Input: part model. Units: mm. Frame: model coordinates. A direction names the side the tool comes from. Give positions to 0.01 mm unless a question says otherwise; leave off trailing zeros. Write each loop counter-clockwise with the first axis right and the second up, starting at its lowest first coordinate (ties: lowest second). Pieces come first, ordered by that corner, then holes. Notation, with made-up numbers: M 7.5,12 L 47.5,12 A31 cw 47.5,47 Z; hole C 63,12.25 d4. An arc over 180 degrees is marked long. Use CSV: the item, a comma, the result in double quotes. Start each with the question number.
from build123d import *

# Parameters (mm, degrees)
F2_R     = 14
F3_DEPTH = 25
F4_SIZE  = 1
F5_R     = 1


with BuildPart() as f1:
    # F0 (on Front) → F1 (revolve)
    with BuildSketch(Plane.XZ):
        Polygon((0, 14), (0, 0), (68, 0), (68, 8), (10, 8), (10, 14), align=None)
    revolve(axis=Axis((34, 0, 0), (1, 0, 0)))

    # F2 (on face) → F3 (cut)
    with BuildSketch(Plane(origin=(0, 0, 0), x_dir=(0, -1, 0), z_dir=(-1, 0, 0))):
        Circle(F2_R)
        Polygon((-12, 6.928203), (0, 13.856406), (12, 6.928203), (12, -6.928203), (0, -13.856406), (-12, -6.928203), align=None, mode=Mode.SUBTRACT)
    extrude(amount=-F3_DEPTH, mode=Mode.SUBTRACT)

    # F4
    f4_edges = [f1.edges().sort_by_distance(p)[0] for p in [
        (68, 0, -8),
    ]]
    chamfer(f4_edges, length=F4_SIZE)

    # F5
    f5_edges = [f1.edges().sort_by_distance(p)[0] for p in [
        (10, 0, -8),
    ]]
    fillet(f5_edges, radius=F5_R)

    # F6 (on Front) → F7 (revolve, cut)
    with BuildSketch(Plane.XZ):
        Polygon((0, 26.713991), (0, 11), (4.210551, 26.713991), align=None)
    revolve(axis=Axis((44.15636, 0, 0), (1, 0, 0)), mode=Mode.SUBTRACT)


solid = f1.part
Q1. First-contact query: pin 1 Ø8 at (x, z) = (17, -1.5) entering from +Y; pin 2 Ø5 at (x, z) = (14.5, -7.5) entering from +Y (3 decimals); pin 3 Ø2 at (x, z) = (12, 3) entering from -Y. Flat tips, straight axial feed; report the tip coordinate or a pass-through.
Q2. Section A-A, the plane z = 0. Return the cut outline in (x, y).
Q3. Material intervals for L1, parallel to X at y = -7.25, z = -5.5; L2, parallel to X at y = -10, z = 5.75; L3, parallel to Y at x = 6.5, z = 10.5, sorted ascending. Write a range as [from, to].
Q4. Set-up query: faces 1 (the cylindrical face through (38.61, 7.81, -1.73)), 2 (the flat face through (5.07, -5.92, 10.44)). Return all of +Z, -Z, +X, -X, +Y, -Y with unobstructed straight access to the full face (end or side cutting, diameter ignored); none if empty.
Q5. Section B-B, the plane x = 7. Return the cut outline in (y, z).
Check result:
1,pin 1,"stops at y = 8"
1,pin 2,"stops at y = 6.245"
1,pin 3,"stops at y = -7.75"
2,outline,"M 0,-11 L 0.27,-12 L 10,-12 L 10,-9 A1 cw 11,-8 L 67,-8 L 68,-7 L 68,7 L 67,8 L 11,8 A1 cw 10,9 L 10,12 L 0.27,12 L 0,11 Z"
3,L1,"x = [0, 10]"
3,L2,"x = [0.14, 10]"
3,L3,"y = [-5.81, 5.81]"
4,face 1,"+X"
4,face 2,"+Z, +X, -X, -Y"
5,outline,"M -12,-6.93 L 0,-13.86 L 12,-6.93 L 12,6.93 L 0,13.86 L -12,6.93 Z"
